Design review of the part built by this model. Coordinates are the model's own, in mm. A direction names the side the tool comes from. Give positions to 0.01 mm unless a question says otherwise; leave off trailing zeros. Write each loop counter-clockwise with the first axis right and the second up, starting at its lowest first coordinate (ties: lowest second). Pieces come first, ordered by that corner, then holes. Notation, with made-up numbers: (81.5, -27) -> (139.5, -27) arc R17 cw to (139.5, -21) -> close; hole circle Ø10 at (15, 37). An arc over 180 degrees is marked (long way). Put each result on its own line as item: value. Start each with the question number.
from build123d import *

# Parameters (mm, degrees)
PAD_DEPTH    = 4
SKETCH001_W  = 4
SKETCH001_H  = 1
PAD001_DEPTH = 1
SKETCH002_W  = 4
SKETCH002_H  = 1
PAD002_DEPTH = 1


with BuildPart() as part:
    # Sketch → Pad (new body)
    with BuildSketch(Plane.XY):
        Polygon((75, 70), (-75, 70), (-75, -70), (75, -70), (75, -2.05), (0, -2.05), (0, 2.05), (75, 2.05), align=None)
    extrude(amount=PAD_DEPTH)

    # Sketch001 (on Face9 of Pad) → Pad001 (join)
    with BuildSketch(Plane(origin=(0, 0, 0), x_dir=(1, 0, 0), z_dir=(0, 0, -1))):
        with Locations((-73, 2.55)):
            Rectangle(SKETCH001_W, SKETCH001_H)
    extrude(amount=PAD001_DEPTH)

    # Sketch002 (on Face4 of Pad001) → Pad002 (join)
    with BuildSketch(Plane(origin=(0, 0, 0), x_dir=(1, 0, 0), z_dir=(0, 0, -1))):
        with Locations((-73, -2.55)):
            Rectangle(SKETCH002_W, SKETCH002_H)
    extrude(amount=PAD002_DEPTH)


solid = part.part
Q1. Take a section at A-A on x = 10.5. Give the boundary of the cut face in (y, z).
Q2. To check wall thickness, follow probe 1 along Y at (x, z) = (48.5, 2.15); probe 2 along Z at (x, y) = (42, -61.5); probe 3 along X at (y, z) = (-2, 1.5). State the ranges of each line that lie inside material, in increasing order. Write a range as from..to.
Q3. Take a section at C-C on y = 54. Give the boundary of the cut face in (x, z), then the cut area to 3 significant figures.
Q4. Mouldability with a two-part tool opening along Y and no side actions: class faces 1 (the face through (37, 2.05, 2)), 2 (the face through (-1, -70, 2)), 3 (the face through (-1, 1, 4)), 4 (the face through (0, 0, 2)) as +Y half, -Y half, draft (parallel to the pull), parting line (faces both ways), or undercut.
Q5. Take a section at B-B on x = -12. Give the boundary of the cut face in (y, z).
Q6. Machinability: for faces 5 (the face through (75, 36, 2)), 6 (the face through (38, -2.05, 2)), which of the approach directions +Z, -Z, +X, -X, +Y, -Y give a long, thin tool a straight path to every point of the face, cutting with its end or side? Answer none if there is none.
Q7. For pin 1 (0.8 mm diameter, centred on x = -72.5, z = -0.5, fed in from +Y); pin 2 (4 mm diameter, centred on x = -32, y = 36, fed in from -Z); pin 3 (1.2 mm diameter, centred on y = 0, z = 1.5, fed in from +X), all flat-tipped, find the tip position at first contact; note any pin that passes through.
Result:
1. outline: (-70, 0) -> (-2.05, 0) -> (-2.05, 4) -> (-70, 4) -> close; (2.05, 0) -> (70, 0) -> (70, 4) -> (2.05, 4) -> close
2. probe 1: y = -70..-2.05, 2.05..70
2. probe 2: z = 0..4
2. probe 3: x = -75..0
3. outline: (-75, 0) -> (75, 0) -> (75, 4) -> (-75, 4) -> close
3. area: 600 mm^2
4. face 1: undercut
4. face 2: -Y half
4. face 3: draft
4. face 4: undercut
5. outline: (-70, 0) -> (70, 0) -> (70, 4) -> (-70, 4) -> close
6. face 5: +Z, -Z, +X, +Y, -Y
6. face 6: +Z, -Z, +X
7. pin 1: stops at y = 3.05
7. pin 2: stops at z = 0
7. pin 3: stops at x = 0
